Design review of the part built by this model. Coordinates are the model's own, in mm. A direction names the side the tool comes from. Round coordinates to 2 decimals unless told otherwise and drop trailing zeros. Order: outer loops, then holes, each group sorted by start corner. A loop starts at its lowest first (then second) coordinate and runs counter-clockwise, first axis right, second up. Notation, with made-up numbers: M -8.75,68 L 42.25,68 A12 ccw 42.25,84 Z; hole C 16.5,-8.5 d4. An arc over 180 degrees is marked long. Use a Markdown table: item, result. Add a question column.
(1) Machinability: for faces 4 (the face through (10.25, -32.36, 8.4)), 5 (the face through (15.875, -28, 3)), 6 (the face through (0, -11, 3.81)), which of the approach directions +Z, -Z, +X, -X, +Y, -Y give a long, thin tool a straight path to every point of the face, cutting with its end or side? Answer none if there is none.
(2) Take a section at B-B (z = 11.5). Write out the cut boundary in (x, y) (3 decimals), then the cut area to 3 significant figures.
(3) For pin 1 (4 mm diameter, centred on x = -13.5, y = -18.5, fed in from +Z); pin 2 (6 mm diameter, centred on x = -9.525, z = 10.16, fed in from +Y); pin 3 (6 mm diameter, centred on x = -11, y = -14.5, fed in from -Z); pin 4 (8 mm diameter, centred on y = 13, z = 2, fed in from +X), all flat-tipped, find the tip position at first contact; note any pin that passes through.
(4) Take a section at D-D (x = -8.5). Write out the cut boundary in (y, z), then the cut area to 3 significant figures.
(5) The part is to be moulded in two halves that separate along X. For faces 1 (the face through (-10.684, -32.358, 8.648)), 2 (the face through (0, -32, 16.51)), 3 (the face through (-15.875, -28, 3)), say which applies: released by +X, released by -X, zero draft, split by the parting line, or undercut.
(6) To check wall thickness, follow probe 1 along X at (y, z) = (-33.5, 10.16) (3 decimals); probe 2 along Z at (x, y) = (5.5, -22.5); probe 3 along Y at (x, z) = (15.5, 1.05). State the ranges of each line that lie inside material, in increasing order. Write a range as from..to.
(7) Take a section at A-A (x = 0). Write out the cut boundary in (y, z).
(8) Take a section at C-C (y = 2.5). Write out the cut boundary in (x, z), then the cut area to 3 significant figures.
```python
from build123d import *

# Parameters (mm, degrees)
BOSS_EXTRUDE1_DEPTH = 3.81
SKETCH3_R           = 7
CUT_EXTRUDE1_DEPTH  = 40.386802358
SKETCH4_W           = 31.75
SKETCH4_H           = 3.81
BOSS_EXTRUDE2_DEPTH = 12.7
SKETCH5_R           = 1.905
CUT_EXTRUDE2_DEPTH  = 56.514417046
SKETCH6_R           = 1.75
CUT_EXTRUDE3_DEPTH  = 42.207937342


with BuildPart() as part:
    # Sketch1 → Boss-Extrude1 (new body)
    with BuildSketch(Plane.XY):
        with BuildLine():
            ThreePointArc((19, 0), (-5.448623679, 18.201991649), (-15.875, -10.43955818))
            Line((-15.875, -10.43955818), (15.875, -10.43955818))
            ThreePointArc((15.875, -10.43955818), (18.201991649, -5.448623679), (19, 0))
        make_face()
        with BuildLine():
            ThreePointArc((15.875, -10.43955818), (0, -19), (-15.875, -10.43955818))
            Line((-15.875, -10.43955818), (-15.875, -34.29))
            Line((-15.875, -34.29), (15.875, -34.29))
            Line((15.875, -34.29), (15.875, -10.43955818))
        make_face()
        with BuildLine():
            Line((15.875, -10.43955818), (-15.875, -10.43955818))
            ThreePointArc((-15.875, -10.43955818), (0, -19), (15.875, -10.43955818))
        make_face()
    extrude(amount=BOSS_EXTRUDE1_DEPTH)

    # Sketch3 → Cut-Extrude1 (cut, through all)
    with BuildSketch(Plane.XY.offset(3.81)):
        Circle(SKETCH3_R)
    extrude(amount=-CUT_EXTRUDE1_DEPTH, mode=Mode.SUBTRACT)

    # Sketch4 → Boss-Extrude2 (add)
    with BuildSketch(Plane.XY.offset(3.81)):
        with Locations((0, -32.385)):
            Rectangle(SKETCH4_W, SKETCH4_H)
    extrude(amount=BOSS_EXTRUDE2_DEPTH)

    # Sketch5 → Cut-Extrude2 (cut, through all)
    with BuildSketch(Plane(origin=(0, -30.48, 0), x_dir=(1, 0, 0), z_dir=(0, 1, 0))):
        with Locations(Location((-9.525, -10.16, 0), (0, 0, 270))):
            Circle(SKETCH5_R)
        with Locations(Location((9.525, -10.16, 0), (0, 0, 90))):
            Circle(SKETCH5_R)
    extrude(amount=-CUT_EXTRUDE2_DEPTH, mode=Mode.SUBTRACT)

    # Sketch6 → Cut-Extrude3 (cut, through all)
    with BuildSketch(Plane.XY.offset(3.81)):
        with Locations((15.5, 0)):
            Circle(SKETCH6_R)
        with Locations((-15.5, 0)):
            Circle(SKETCH6_R)
    extrude(amount=-CUT_EXTRUDE3_DEPTH, mode=Mode.SUBTRACT)


solid = part.part
```
Verdict:
| question | item | result |
|---|---|---|
| 1 | face 4 | +Y, -Y |
| 1 | face 5 | +Z, -Z, +X, -Y |
| 1 | face 6 | +Z, +X, -X, +Y |
| 2 | outline | M -15.875,-34.29 L -10.879,-34.29 L -10.879,-30.48 L -15.875,-30.48 Z; M -8.171,-34.29 L 8.171,-34.29 L 8.171,-30.48 L -8.171,-30.48 Z; M 10.879,-34.29 L 15.875,-34.29 L 15.875,-30.48 L 10.879,-30.48 Z |
| 2 | area | 100 mm^2 |
| 3 | pin 1 | stops at z = 3.81 |
| 3 | pin 2 | stops at y = -30.48 |
| 3 | pin 3 | stops at z = 0 |
| 3 | pin 4 | stops at x = 16.73 |
| 4 | outline | M -34.29,0 L 16.99,0 L 16.99,3.81 L -30.48,3.81 L -30.48,8.55 L -34.29,8.55 Z; M -34.29,11.77 L -30.48,11.77 L -30.48,16.51 L -34.29,16.51 Z |
| 4 | area | 232 mm^2 |
| 5 | face 1 | undercut |
| 5 | face 2 | zero draft |
| 5 | face 3 | released by -X |
| 6 | probe 1 | x = -15.875..-11.43, -7.62..7.62, 11.43..15.875 |
| 6 | probe 2 | z = 0..3.81 |
| 6 | probe 3 | y = -34.29..-1.75, 1.75..10.99 |
| 7 | outline | M -34.29,0 L -7,0 L -7,3.81 L -30.48,3.81 L -30.48,16.51 L -34.29,16.51 Z; M 7,0 L 19,0 L 19,3.81 L 7,3.81 Z |
| 8 | outline | M -18.83,0 L -6.54,0 L -6.54,3.81 L -18.83,3.81 Z; M 6.54,0 L 18.83,0 L 18.83,3.81 L 6.54,3.81 Z |
| 8 | area | 93.7 mm^2 |
